Geometry check sheet. Reference: the model listing, model coordinates, mm. Face numbers are marked on the shaded views. Round coordinates to 2 decimals unless told otherwise and drop trailing zeros. Write each loop counter-clockwise with the first axis right and the second up, starting at its lowest first coordinate (ties: lowest second). Pieces come first, ordered by that corner, then holes. Notation, with made-up numbers: M 45.5,-14 L 59.5,-14 A14 cw 59.5,10 Z; hole C 80,73.25 d10. An arc over 180 degrees is marked long. Use a Markdown table: item, result.
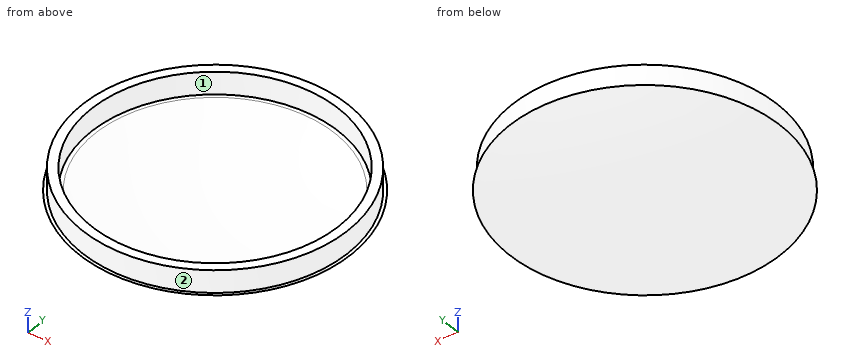
```python
from build123d import *

# Parameters (mm, degrees)
F3_T     = -1.27
F4_W     = 834.6531093121
F4_H     = 674.1969883442
F5_DEPTH = 508
F0_R     = 37.211
F0_R_2   = 34.671
F6_DEPTH = 6.35


with BuildPart() as f2:
    # F1 (on Front) → F2 (revolve)
    with BuildSketch(Plane.XZ):
        with BuildLine():
            ThreePointArc((127, 121.158), (0, 248.158), (-127, 121.158))
            Line((-127, 121.158), (127, 121.158))
        make_face()
    revolve(axis=Axis((0, 0, 121.158), (1, 0, 0)))

    # F3 (hollow: no face is removed)
    offset(amount=F3_T, mode=Mode.SUBTRACT)

    # F4 (on Top) → F5 (cut)
    with BuildSketch(Plane.XY):
        with Locations((43.5875803232, -34.0506881475)):
            Rectangle(F4_W, F4_H)
    extrude(amount=F5_DEPTH, mode=Mode.SUBTRACT)

    # F0 (on Top) → F6 (join)
    with BuildSketch(Plane.XY):
        Circle(F0_R)
        Circle(F0_R_2, mode=Mode.SUBTRACT)
    extrude(amount=F6_DEPTH)


solid = f2.part
```
Item 1: Go/stop test with flat-tipped pins: pin 1 (1 mm diameter, centred on y = 15.5, z = 4.5, fed in from -X); pin 2 (6 mm diameter, centred on x = -8, y = -5.5, fed in from +Z); pin 3 (1.5 mm diameter, centred on x = -25, y = 14.5, fed in from +Z). Record where each tip stops, or that it passes through.
Outcome:
| item | result |
|---|---|
| pin 1 | stops at x = -34.05 |
| pin 2 | stops at z = -3.93 |
| pin 3 | stops at z = -1.03 |
Item 2: Material ranges on line 1 along Y through (x, z) = (0, 4.5); line 2 along X through (y, z) = (-23, 2.25); line 3 along X through (y, z) = (14, 0.5), recorded low to high. Write a range as from..to.
Outcome:
| item | result |
|---|---|
| line 1 | y = -37.21..-34.67, 34.67..37.21 |
| line 2 | x = -29.25..-25.94, 25.94..29.25 |
| line 3 | x = -34.48..-31.72, 31.72..34.48 |
Item 3: Cross-section at A-A, the plane x = 0. Record the cut outline in (y, z), and give its area (3 significant figures).
Outcome:
| item | result |
|---|---|
| outline | M -38.08,0 A127 ccw 38.08,0 L 37.21,0 L 37.21,6.35 L 34.67,6.35 L 34.67,0 L 33.6,0 A125.73 cw -33.6,0 L -34.67,0 L -34.67,6.35 L -37.21,6.35 L -37.21,0 Z |
| area | 125 mm2 |
Item 4: Cross-section at C-C, the plane z = 2. Record the cut outline in (x, y), and give its area (3 significant figures).
Outcome:
| item | result |
|---|---|
| outline | C 0,0 d74.42; hole C 0,0 d69.34 |
| area | 574 mm2 |
Item 5: Cross-section at B-B, the plane y = -20. Record the cut outline in (x, z).
Outcome:
| item | result |
|---|---|
| outline | M -32.4,0 A125.42 ccw 32.4,0 L 31.38,0 L 31.38,6.35 L 28.32,6.35 L 28.32,0 L 27,0 A124.13 cw -27,0 L -28.32,0 L -28.32,6.35 L -31.38,6.35 L -31.38,0 Z |
Item 6: Mould release check, pull along X, two halves, no side actions. Record for the marked faces 1 and 2: +X half, -X half, draft (parallel to the pull), parting line (faces both ways), or undercut.
Outcome:
| item | result |
|---|---|
| face 1 | undercut |
| face 2 | parting line |
